Input: part model. Units: mm. Frame: model coordinates. A direction names the side the tool comes from. Give positions to 0.01 mm unless a question says otherwise; leave off trailing zeros. Loops run counter-clockwise (first coordinate to the right, second up) from the corner with the lowest first, then second, coordinate; pieces in that order, holes last. Notation, with made-up numbers: (-40, 62) -> (-26, 62) arc R5 cw to (-26, 70) -> close; hole circle Ø9 at (50.25, 58). An arc over 180 degrees is marked (long way). Use CSV: the item, a comma, the result in double quotes.
```python
from build123d import *

# Parameters (mm, degrees)
F0_W     = 5
F0_H     = 10
F1_DEPTH = 2.5
F2_R     = 2
F3_DEPTH = 12.5
F4_R     = 2
F5_DEPTH = 7.5


with BuildPart() as f1:
    # F0 (on Top) → F1 (new body, symmetric)
    with BuildSketch(Plane.XY):
        Rectangle(F0_W, F0_H)
    extrude(amount=F1_DEPTH, both=True)

    # F2 (on Front) → F3 (join, symmetric)
    with BuildSketch(Plane.XZ):
        Circle(F2_R)
    extrude(amount=F3_DEPTH, both=True)

    # F4 (on Right) → F5 (join, symmetric)
    with BuildSketch(Plane.YZ):
        Circle(F4_R)
    extrude(amount=F5_DEPTH, both=True)


solid = f1.part
```
1) Section query C-C (y = 0). Return loops of the section in (x, z).
From the geometry:
outline,"(-7.5, -2) -> (-2.5, -2) -> (-2.5, -2.5) -> (2.5, -2.5) -> (2.5, -2) -> (7.5, -2) -> (7.5, 2) -> (2.5, 2) -> (2.5, 2.5) -> (-2.5, 2.5) -> (-2.5, 2) -> (-7.5, 2) -> close"
2) Section query B-B (z = 0). Return loops of the section in (x, y).
From the geometry:
outline,"(-7.5, -2) -> (-2.5, -2) -> (-2.5, -5) -> (-2, -5) -> (-2, -12.5) -> (2, -12.5) -> (2, -5) -> (2.5, -5) -> (2.5, -2) -> (7.5, -2) -> (7.5, 2) -> (2.5, 2) -> (2.5, 5) -> (2, 5) -> (2, 12.5) -> (-2, 12.5) -> (-2, 5) -> (-2.5, 5) -> (-2.5, 2) -> (-7.5, 2) -> close"
3) Contact query for flat-ended pins moving along their axis: pin 1 (3 mm diameter, centred on y = 3.5, z = -0.5, fed in from +X); pin 2 (3 mm diameter, centred on y = -10, z = 1.5, fed in from -X). Output: stop coordinate, or through.
From the geometry:
pin 1,"stops at x = 2.5"
pin 2,"stops at x = -2"
4) Ray query, line 1 (Y direction, x = -1.5, z = -2.1); line 2 (X direction, y = -7.5, z = 0.1); line 3 (X direction, y = 5.5, z = -0.5). Return the intervals inside material, ascending.
From the geometry:
line 1,"y = -5 to 5"
line 2,"x = -2 to 2"
line 3,"x = -1.94 to 1.94"
5) Section query A-A (x = 0). Return loops of the section in (y, z), then the cut area to 3 significant figures.
From the geometry:
outline,"(-12.5, -2) -> (-5, -2) -> (-5, -2.5) -> (5, -2.5) -> (5, -2) -> (12.5, -2) -> (12.5, 2) -> (5, 2) -> (5, 2.5) -> (-5, 2.5) -> (-5, 2) -> (-12.5, 2) -> close"
area,"110 mm^2"
6) Reachability of faces 1 (the cylindrical face through (5, 0, -2)), 2 (the cylindrical face through (0, 9, -2)), 3 (the flat face through (-1, -5, 2)), 4 (the cylindrical face through (-5, 0, -2)), 5 (the flat face through (0, 12.5, 0)) from +Z, -Z, +X, -X, +Y, -Y: full face, straight path, thin tool, end or side. Return the list, or none.
From the geometry:
face 1,"+X"
face 2,"+Y"
face 3,"-Y"
face 4,"-X"
face 5,"+Z, -Z, +X, -X, +Y"
7) Section query D-D (y = 3.25). Return loops of the section in (x, z), then the cut area to 3 significant figures.
From the geometry:
outline,"(-2.5, -2.5) -> (2.5, -2.5) -> (2.5, 2.5) -> (-2.5, 2.5) -> close"
area,"25.0 mm^2"
